Read the model definition and answer for the solid it produces. Units are mm, in the model's axes. Face numbers are marked on the shaded views. Coordinates: 2 decimals unless noted, no trailing zeros. Order: outer loops, then holes, each group sorted by start corner. A loop starts at its lowest first (then second) coordinate and runs counter-clockwise, first axis right, second up. Notation, with made-up numbers: (3, 21.5) -> (53, 21.5) arc R25 ccw to (53, 46.5) -> close; hole circle Ø7 at (43, -5.75). An arc over 180 degrees is marked (long way). Answer as a JSON object with one key per item and string values. Group by question number.
1) Given pin 1 (1 mm diameter, centred on y = 169, z = 0.5, fed in from +X), flat-ended and moving along its own axis, determine where the tip first touches the part or whether it passes through.
2) Section B-B on x = 54.5 is taken. Determine the outline of the cut face in (y, z) (3 decimals), and give its area (3 significant figures).
3) Section C-C on y = 78 is taken. Determine the outline of the cut face in (x, z) (3 decimals), and give its area (3 significant figures).
4) Consider L1, parallel to Y at x = 0.5, z = 0.6 (3 decimals); L2, parallel to Y at x = 50.5, z = 1.5 (3 decimals); L3, parallel to X at y = 215.9, z = 0.9 (3 decimals). Determine where each line is inside the solid, lowest interval first.
5) Section A-A on z = 2.65 is taken. Determine the outline of the cut face in (x, y) (3 decimals), and give its area (3 significant figures).
6) Determine the mould class of the marked faces 1 and 2 for opening direction Z: released by +Z, released by -Z, zero draft, split by the parting line, or undercut.
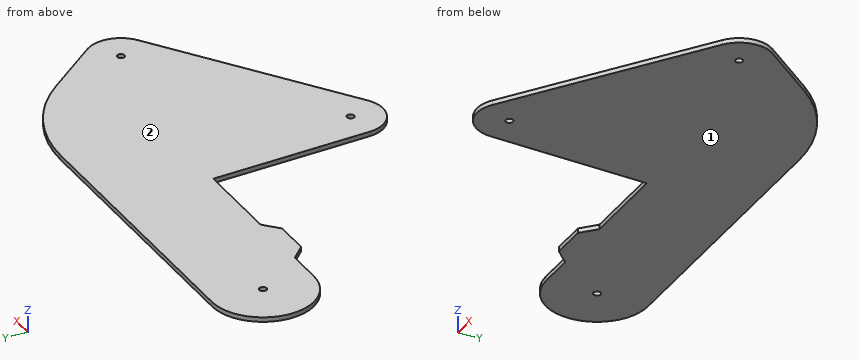
from build123d import *

# Parameters (mm, degrees)
SKETCH1_R           = 2.54
BOSS_EXTRUDE1_DEPTH = 3.175


with BuildPart() as part:
    # Sketch1 → Boss-Extrude1 (new body)
    with BuildSketch(Plane.XY):
        with BuildLine():
            Line((134.62, 180.975), (142.401211704, 69.698488351))
            ThreePointArc((142.401211704, 69.698488351), (155.003963594, 51.188868036), (177.319809019, 53.043171796))
            Line((177.319809019, 53.043171796), (307.36019605, 144.098431067))
            ThreePointArc((307.36019605, 144.098431067), (316.647321796, 159.403140629), (311.6377975, 176.590039876))
            Line((311.6377975, 176.590039876), (279.800527192, 214.532221144))
            ThreePointArc((279.800527192, 214.532221144), (244.908427164, 241.305871163), (201.970411771, 250.825))
            Line((201.970411771, 250.825), (0, 250.825))
            ThreePointArc((0, 250.825), (-34.925, 215.9), (0, 180.975))
            Line((0, 180.975), (25.4, 180.975))
            Line((25.4, 180.975), (35.56, 171.45))
            Line((35.56, 171.45), (60.96, 171.45))
            Line((60.96, 171.45), (71.12, 180.975))
            Line((71.12, 180.975), (134.62, 180.975))
        make_face()
        with Locations((294.612459752, 162.304085251)):
            Circle(SKETCH1_R, mode=Mode.SUBTRACT)
        with Locations((164.572072721, 71.24882598)):
            Circle(SKETCH1_R, mode=Mode.SUBTRACT)
        with Locations((0, 215.9)):
            Circle(SKETCH1_R, mode=Mode.SUBTRACT)
    extrude(amount=BOSS_EXTRUDE1_DEPTH)


solid = part.part
Worked answers:
{
 "1": {"pin 1": "stops at x = 315.96"},
 "2": {"outline": "(171.45, 0) -> (250.825, 0) -> (250.825, 3.175) -> (171.45, 3.175) -> close", "area": "252 mm²"},
 "3": {"outline": "(141.821, 0) -> (212.962, 0) -> (212.962, 3.175) -> (141.821, 3.175) -> close", "area": "226 mm²"},
 "4": {"L1": "y = 180.975 to 213.41, 218.39 to 250.825", "L2": "y = 171.45 to 250.825", "L3": "x = -34.925 to -2.54, 2.54 to 278.632"},
 "5": {"outline": "(0, 180.975) -> (25.4, 180.975) -> (35.56, 171.45) -> (60.96, 171.45) -> (71.12, 180.975) -> (134.62, 180.975) -> (142.401, 69.698) arc R22.225 ccw to (177.32, 53.043) -> (307.36, 144.098) arc R22.225 ccw to (311.638, 176.59) -> (279.801, 214.532) arc R101.6 ccw to (201.97, 250.825) -> (0, 250.825) arc R34.925 ccw to start; hole circle Ø5.08 at (0, 215.9); hole circle Ø5.08 at (164.572, 71.249); hole circle Ø5.08 at (294.612, 162.304)", "area": "37,200 mm²"},
 "6": {"face 1": "released by -Z", "face 2": "released by +Z"}
}
